from build123d import *

# Parameters (mm, degrees)
F0_W     = 381
F0_H     = 381
F1_DEPTH = 9.525
F2_W     = 69.85
F2_H     = 69.85
F3_DEPTH = 9.525
F4_R     = 3.175


with BuildPart() as f1:
    # F0 (on Top) → F1 (new body)
    with BuildSketch(Plane.XY):
        with Locations((190.5, 190.5)):
            Rectangle(F0_W, F0_H)
    extrude(amount=F1_DEPTH)

    # F2 (on face) → F3 (cut, through all)
    with BuildSketch(Plane.XY.offset(9.525)):
        with Locations((73.025, 73.025)):
            Rectangle(F2_W, F2_H)
    extrude(amount=-F3_DEPTH, mode=Mode.SUBTRACT)

    # F4
    f4_edges = [f1.edges().sort_by_distance(p)[0] for p in [
        (0, 190.5, 0),
        (190.5, 0, 0),
        (381, 190.5, 0),
        (190.5, 381, 0),
    ]]
    fillet(f4_edges, radius=F4_R)


solid = f1.part
Geometry check sheet. Reference: the model listing, model coordinates, mm. A direction names the side the tool comes from. Give positions to 0.01 mm unless a question says otherwise; leave off trailing zeros. Loops run counter-clockwise (first coordinate to the right, second up) from the corner with the lowest first, then second, coordinate; pieces in that order, holes last. Notation, with made-up numbers: M -5.75,-32.75 L 2.25,-32.75 A18 cw 2.25,-22.75 Z; hole C -16.75,-6.75 d5. An arc over 180 degrees is marked long. Answer as a JSON object with one key per item and string values. Group by question number.
Item 1: Sectioned sample at C-C on z = 6.5. Record the boundary of the cut face in (x, y), plus the area to 3 significant figures.
Item 2: Access from +Z, -Z, +X, -X, +Y, -Y to the whole of each face (thin tool, end or side, straight path). Record for faces 1 (the flat face through (73, 107.95, 5)), 2 (the flat face through (188, 193, 9.525)).
Item 3: Mould release check, pull along Y, two halves, no side actions. Record for faces 3 (the flat face through (107.95, 73, 5)), 4 (the flat face through (188, 193, 0)): pulls with the +Y half, pulls with the -Y half, needs draft (parallel to the pull), parting line crosses it, or undercut.
Item 4: Sectioned sample at A-A on y = 98. Record the boundary of the cut face in (x, z) (3 decimals), plus the area to 3 significant figures.
Item 5: Gauge pin test, flat end, axial feed: pin 1 (1 mm diameter, centred on x = 310.5, z = 2.5, fed in from +Y). Record the tip position at first contact, or that the pin passes through.
Item 6: Material ranges on L1, parallel to X at y = 99.5, z = 4.5; L2, parallel to X at y = 189.5, z = 2.75; L3, parallel to Y at x = 210.5, z = 1.25, recorded low to high.
Findings below:
{
 "1": {"outline": "M 0,0 L 381,0 L 381,381 L 0,381 Z; hole M 38.1,38.1 L 107.95,38.1 L 107.95,107.95 L 38.1,107.95 Z", "area": "140,000 mm2"},
 "2": {"face 1": "+Z, -Z", "face 2": "+Z, +X, -X, +Y, -Y"},
 "3": {"face 3": "undercut", "face 4": "needs draft"},
 "4": {"outline": "M 0,3.175 A3.175 ccw 3.175,0 L 38.1,0 L 38.1,9.525 L 0,9.525 Z; M 107.95,0 L 377.825,0 A3.175 ccw 381,3.175 L 381,9.525 L 107.95,9.525 Z", "area": "2,960 mm2"},
 "5": {"pin 1": "y = 381"},
 "6": {"L1": "0 to 38.1, 107.95 to 381", "L2": "0.03 to 380.97", "L3": "0.65 to 380.35"}
}
